The model under review builds one solid part; all positions refer to its coordinate system, in mm. Round coordinates to 2 decimals unless told otherwise and drop trailing zeros. Order: outer loops, then holes, each group sorted by start corner. A loop starts at its lowest first (then second) coordinate and runs counter-clockwise, first axis right, second up. Notation, with made-up numbers: (-18, -27.75) -> (16, -27.75) arc R21 ccw to (16, -2.75) -> close; hole circle Ø5 at (-35.5, 68). An arc over 180 degrees is marked (long way). Use a Markdown table: item, result. Add a question column.
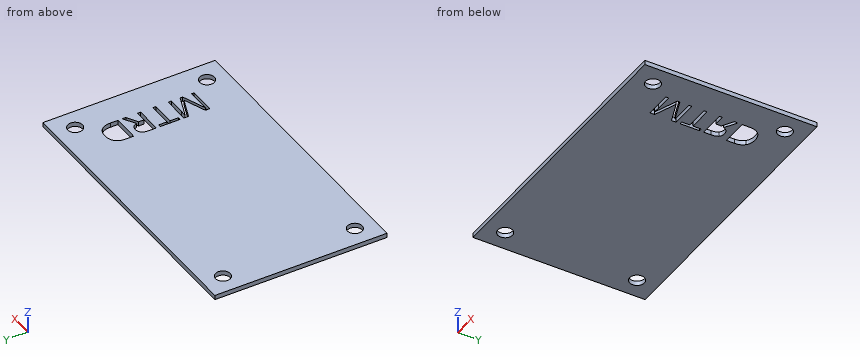
```python
from build123d import *

# Parameters (mm, degrees)
F0_W     = 63.5
F0_H     = 38.11
F0_R     = 1.63195
F1_DEPTH = 1


with BuildPart() as f1:
    # F0 (on Top) → F1 (new body)
    with BuildSketch(Plane.XY):
        Rectangle(F0_W, F0_H)
        with Locations((-27.305, -14.605)):
            Circle(F0_R, mode=Mode.SUBTRACT)
        with Locations((27.305, -14.605)):
            Circle(F0_R, mode=Mode.SUBTRACT)
        with BuildLine():
            Line((25.0343345106, -7.2836339695), (25.0343345106, -7.8282632467))
            Line((25.0343345106, -7.8282632467), (19.8807163504, -9.800635629))
            Line((19.8807163504, -9.800635629), (19.8807163504, -9.8324480867))
            add(Edge.make_bspline(
                [(19.8807163504, -9.8324480867), (20.4927880381, -9.776458161), (21.3364544184, -9.776458161)],
                knots=[0, 0, 0, 1, 1, 1], degree=2))
            Line((21.3364544184, -9.776458161), (25.0343345106, -9.776458161))
            Line((25.0343345106, -9.776458161), (25.0343345106, -10.4012548318))
            Line((25.0343345106, -10.4012548318), (19.220289727, -10.4012548318))
            Line((19.220289727, -10.4012548318), (19.220289727, -9.3832561829))
            Line((19.220289727, -9.3832561829), (24.0163358617, -7.5419511267))
            Line((24.0163358617, -7.5419511267), (24.0163358617, -7.5101386689))
            Line((24.0163358617, -7.5101386689), (19.220289727, -5.6535636329))
            Line((19.220289727, -5.6535636329), (19.220289727, -4.6431999739))
            Line((19.220289727, -4.6431999739), (25.0343345106, -4.6431999739))
            Line((25.0343345106, -4.6431999739), (25.0343345106, -5.3188965771))
            Line((25.0343345106, -5.3188965771), (21.2880994826, -5.3188965771))
            add(Edge.make_bspline(
                [(21.2880994826, -5.3188965771), (20.6442153371, -5.3188965771), (19.8883513403, -5.2629066514)],
                knots=[0, 0, 0, 1, 1, 1], degree=2))
            Line((19.8883513403, -5.2629066514), (19.8883513403, -5.2947191092))
            Line((19.8883513403, -5.2947191092), (25.0343345106, -7.2836339695))
        make_face(mode=Mode.SUBTRACT)
        Polygon((19.8209089298, -1.2596269646), (25.0343345106, -1.2596269646), (25.0343345106, -1.9353235678), (19.8209089298, -1.9353235678), (19.8209089298, -3.776628624), (19.220289727, -3.776628624), (19.220289727, 0.5816780917), (19.8209089298, 0.5816780917), align=None, mode=Mode.SUBTRACT)
        with Locations((-27.305, 14.605)):
            Circle(F0_R, mode=Mode.SUBTRACT)
        with BuildLine():
            Line((22.6165877194, 3.3468169218), (22.6165877194, 2.1328535329))
            Line((22.6165877194, 2.1328535329), (25.0343345106, 2.1328535329))
            Line((25.0343345106, 2.1328535329), (25.0343345106, 1.4571569297))
            Line((25.0343345106, 1.4571569297), (19.220289727, 1.4571569297))
            Line((19.220289727, 1.4571569297), (19.220289727, 3.0515973136))
            add(Edge.make_bspline(
                [(19.220289727, 3.0515973136), (19.220289727, 4.1217683933), (19.6300341831, 4.6326764652)],
                knots=[0, 0, 0, 1, 1, 1], degree=2))
            add(Edge.make_bspline(
                [(19.6300341831, 4.6326764652), (20.0397786393, 5.1435845371), (20.8630850466, 5.1435845371)],
                knots=[0, 0, 0, 1, 1, 1], degree=2))
            add(Edge.make_bspline(
                [(20.8630850466, 5.1435845371), (22.0159685165, 5.1435845371), (22.4218954778, 3.9741585892)],
                knots=[0, 0, 0, 1, 1, 1], degree=2))
            Line((22.4218954778, 3.9741585892), (25.0343345106, 5.5533289933))
            Line((25.0343345106, 5.5533289933), (25.0343345106, 4.7542000539))
            Line((25.0343345106, 4.7542000539), (22.6165877194, 3.3468169218))
        make_face(mode=Mode.SUBTRACT)
        with BuildLine():
            add(Edge.make_bspline(
                [(19.9716999797, 10.3805513366), (20.7231102324, 11.1319615894), (22.0719584422, 11.1319615894)],
                knots=[0, 0, 0, 1, 1, 1], degree=2))
            add(Edge.make_bspline(
                [(22.0719584422, 11.1319615894), (23.5111540321, 11.1319615894), (24.2727442713, 10.3506476263)],
                knots=[0, 0, 0, 1, 1, 1], degree=2))
            add(Edge.make_bspline(
                [(24.2727442713, 10.3506476263), (25.0343345106, 9.5693336633), (25.0343345106, 8.1021431105)],
                knots=[0, 0, 0, 1, 1, 1], degree=2))
            Line((25.0343345106, 8.1021431105), (25.0343345106, 6.4911602486))
            Line((25.0343345106, 6.4911602486), (19.220289727, 6.4911602486))
            Line((19.220289727, 6.4911602486), (19.220289727, 8.2726578842))
            add(Edge.make_bspline(
                [(19.220289727, 8.2726578842), (19.220289727, 9.6291410839), (19.9716999797, 10.3805513366)],
                knots=[0, 0, 0, 1, 1, 1], degree=2))
        make_face(mode=Mode.SUBTRACT)
        with Locations((27.305, 14.605)):
            Circle(F0_R, mode=Mode.SUBTRACT)
    extrude(amount=F1_DEPTH)


solid = f1.part
```
Q1. Wall thickness on line 1 (X direction, y = 14.5, z = 0.2); line 2 (X direction, y = 8.5, z = 0.1); line 3 (Y direction, x = 28.5, z = 0.85) (3 decimals): over which ranges is each line inside the solid? List them lowest first. Write a range as [from, to].
Q2. Add section B-B (x = 28). Write out the cut boundary in (y, z) (3 decimals), then the cut area to 3 significant figures.
Q3. Add section A-A (x = -26.5). Write out the cut boundary in (y, z) (3 decimals), then the cut area to 3 significant figures.
Q4. Add section C-C (z = 0.3). State how many separate pieces and enclosed holes the cut face has, then the cut area to 3 significant figures.
Report:
| question | item | result |
|---|---|---|
| 1 | line 1 | x = [-31.75, -28.93], [-25.68, 25.68], [28.93, 31.75] |
| 1 | line 2 | x = [-31.75, 19.23], [25.02, 31.75] |
| 1 | line 3 | y = [-19.055, -15.716], [-13.494, 13.494], [15.716, 19.055] |
| 2 | outline | (-19.055, 0) -> (-16.082, 0) -> (-16.082, 1) -> (-19.055, 1) -> close; (-13.128, 0) -> (13.128, 0) -> (13.128, 1) -> (-13.128, 1) -> close; (16.082, 0) -> (19.055, 0) -> (19.055, 1) -> (16.082, 1) -> close |
| 2 | area | 32.2 mm² |
| 3 | outline | (-19.055, 0) -> (-16.025, 0) -> (-16.025, 1) -> (-19.055, 1) -> close; (-13.185, 0) -> (13.185, 0) -> (13.185, 1) -> (-13.185, 1) -> close; (16.025, 0) -> (19.055, 0) -> (19.055, 1) -> (16.025, 1) -> close |
| 3 | area | 32.4 mm² |
| 4 | separate pieces | 1 |
| 4 | enclosed holes | 8 |
| 4 | area | 2,330 mm² |
